Verification items for this drawing (mm, ordinates from the low corner). Give positions to 0.01 mm unless a question says otherwise; leave off trailing zeros. Loops run counter-clockwise (first coordinate to the right, second up) from the corner with the lowest first, then second, coordinate; pieces in that order, holes last. Notation, with made-up numbers: (53.5, 62) -> (75.5, 62) arc R10 ccw to (75.5, 69) -> close; hole circle Ø9 at (4.25, 70). An arc over 180 degrees is marked (long way). Write each question's results on one line, items separated by ' | '. Start each with the question number.
Item 1: Mould release check, pull along Z, two halves, no side actions. Record for the marked faces 1, 2 and 3: pulls with the +Z half, pulls with the -Z half, needs draft (parallel to the pull), parting line crosses it, or undercut.
Item 2: Cross-section at B-B on z = 5.5. Enter the section's corners in (x, y) (1 decimal), then the cut area to 3 significant figures.
Item 3: Cross-section at A-A on x = 9. Enter the section's corners in (y, z) (1 decimal), then the cut area to 3 significant figures.
Item 4: Scan line: line 1 along Y through (x, z) = (15.75, 3). Record every from-to range of solid material in increasing order.
Item 5: Gauge pin test, flat end, axial feed: pin 1 Ø4.5 at (x, z) = (15, 4) entering from +Y. Record the tip position at first contact, or that the pin passes through.
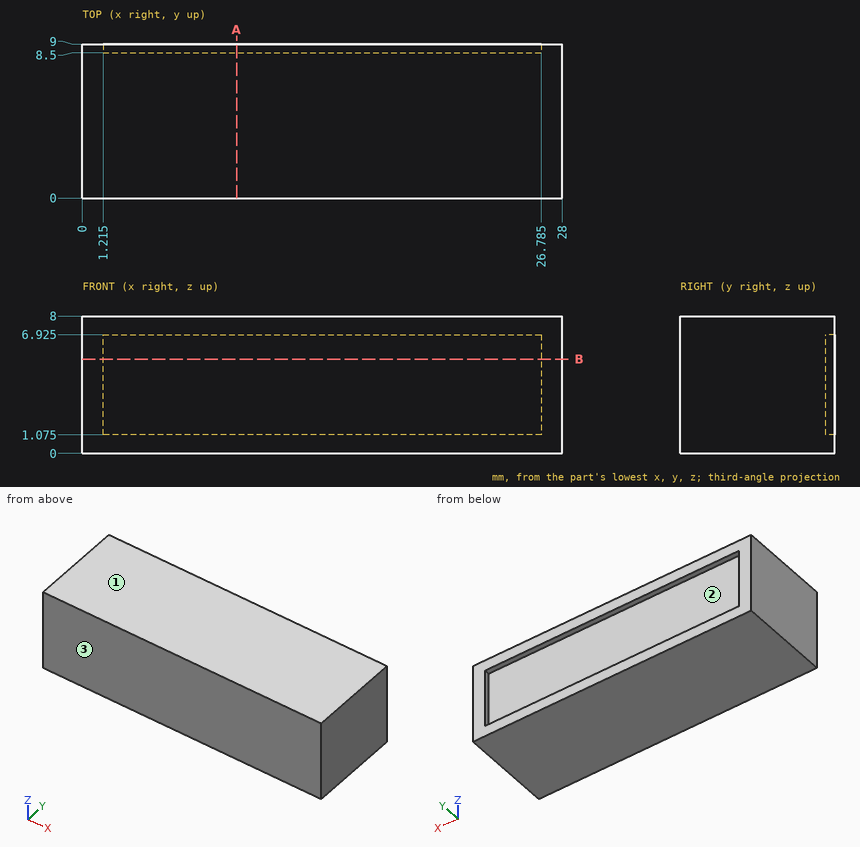
Answer sheet:
1) face 1: pulls with the +Z half | face 2: undercut | face 3: needs draft
2) outline: (0, 0) -> (28, 0) -> (28, 9) -> (26.8, 9) -> (26.8, 8.5) -> (1.2, 8.5) -> (1.2, 9) -> (0, 9) -> close | area: 239 mm²
3) outline: (0, 0) -> (9, 0) -> (9, 1.1) -> (8.5, 1.1) -> (8.5, 6.9) -> (9, 6.9) -> (9, 8) -> (0, 8) -> close | area: 69.1 mm²
4) line 1: y = 0 to 8.5
5) pin 1: stops at y = 8.5
